Solid Edge part; units mm, degrees
sketch "Sketch1" plane through (0, 0, 0) normal (0, 0, 1) x (1, 0, 0)
  line L0 (0, 0) -> (-100, 0)
  line L1 (-100, 0) -> (-100, -94.1)
  line L2 (-100, -94.1) -> (0, -94.1)
  line L3 (0, -94.1) -> (0, 0)
extrude "Protrusion1" add sketch "Sketch1" against normal blind 20
sketch "Sketch2" plane through (-50, -47.05, 0) normal (0, 0, 1) x (1, 0, 0)
  circle A0 centre (-14.73, -7.95) radius 6.7
  circle A1 centre (72.77, -7.95) radius 55
extrude "ExtrudedCutout_1" cut sketch "Sketch2" against normal blind 20
fillet "Round_2" radius 4 1 edges at (0, 0, -10)
fillet "Round_4" radius 1 1 edges at (-15.9106, -94.1, -10)
The listing builds one solid part. Answer for the finished solid, in the listing's coordinates (mm). Give positions to 0.01 mm unless a question says otherwise; leave off trailing zeros. Loops run counter-clockwise (first coordinate to the right, second up) from the corner with the lowest first, then second, coordinate; pieces in that order, holes last.
Item 1: This flat-tipped pin is pushed along its axis until it touches: pin 1 Ø5 at (x, z) = (-79.5, -13.5) entering from +Y. Where does it stop, or does it pass through?
Derived:
pin 1: stops at y = 0
Item 2: A cutting plane is placed at D-D (y = -36). Give the vertices of the cut face in (x, z), then the cut area to 3 significant figures.
Derived:
outline: (-100, -20) - (-28.84, -20) - (-28.84, 0) - (-100, 0) - close
area: 1,420 mm2
Item 3: A cutting plane is placed at A-A (x = -64.73). Give the vertices of the cut face in (y, z).
Derived:
outline: (-94.1, -20) - (-61.7, -20) - (-61.7, 0) - (-94.1, 0) - close; (-48.3, -20) - (0, -20) - (0, 0) - (-48.3, 0) - close
Item 4: Determine the mould class of faces 1 (the flat face through (-62, -46, 0)), 2 (the flat face through (-100, -46, -10)), 3 (the cylindrical face through (-61.13, -49.35, -9.86)) for opening direction X: +X half, -X half, draft (parallel to the pull), parting line (faces both ways), or undercut.
Derived:
face 1: draft
face 2: -X half
face 3: undercut
Item 5: A cutting plane is placed at C-C (z = -12.75). Give the vertices of the cut face in (x, y), then the cut area to 3 significant figures.
Derived:
outline: (-100, -94.1) - (-18.27, -94.1) arc R1 ccw to (-17.54, -92.42) arc R55 cw to (0, -4.93) - (0, -4) arc R4 ccw to (-4, 0) - (-100, 0) - close; hole circle Ø13.4 at (-64.73, -55)
area: 7,040 mm2
Item 6: Find the intervals of material crossed by line 1 along Y through (x, z) = (-64.73, -14); line 2 along Y through (x, z) = (-61.5, -0.75); line 3 along X through (y, z) = (-49.5, -7.5), in increasing order.
Derived:
line 1: y = -94.1 to -61.7, -48.3 to 0
line 2: y = -94.1 to -60.87, -49.13 to 0
line 3: x = -100 to -68.56, -60.9 to -31.95
Item 7: A cutting plane is placed at B-B (y = -55). Give the vertices of the cut face in (x, z), then the cut area to 3 significant figures.
Derived:
outline: (-100, -20) - (-71.43, -20) - (-71.43, 0) - (-100, 0) - close; (-58.03, -20) - (-32.23, -20) - (-32.23, 0) - (-58.03, 0) - close
area: 1,090 mm2
